CAD build for the part. Positions are in the model's coordinates, mm. Round coordinates to 2 decimals unless told otherwise and drop trailing zeros. Write each loop counter-clockwise with the first axis right and the second up, starting at its lowest first coordinate (ties: lowest second). Pieces come first, ordered by that corner, then holes. Notation, with made-up numbers: (34, -37) -> (55, -37) arc R32 ccw to (55, 0) -> close; hole circle Ø8 at (6.5, 49). An arc over 180 degrees is marked (long way). Answer in a Markdown table with one row per item. Add a question column.
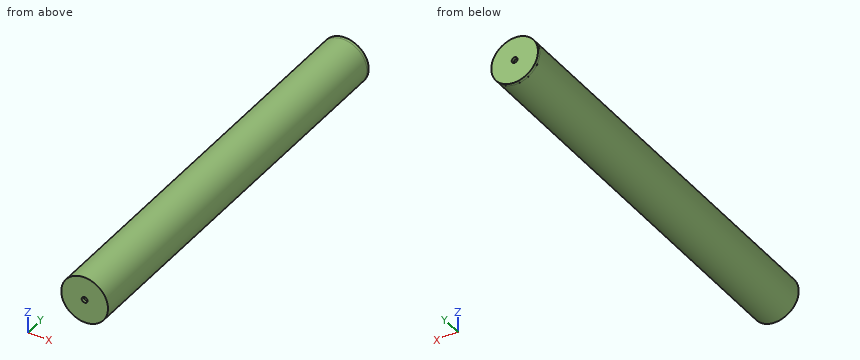
Autodesk Inventor part; units mm, degrees
ref_plane "YZ Plane" through (0, 0, 0) normal (1, 0, 0) x (0, 1, 0)
ref_plane "XZ Plane" through (0, 0, 0) normal (0, 1, 0) x (-1, 0, 0)
ref_plane "XY Plane" through (0, 0, 0) normal (0, 0, 1) x (1, 0, 0)
sketch "Sketch1" plane through (0, 0, 0) normal (0, 1, 0) x (-1, 0, 0)
  circle A0 centre (0, 0) radius 25.4
  circle A1 centre (0, 0) radius 3.175
  dimension "d0" = 50.8
  dimension "d1" = 6.35
extrude "Extrusion1" add sketch "Sketch1" along normal blind 3.175
sketch "Sketch2" plane through (0, 3.175, 0) normal (0, 1, 0) x (1, 0, 0)
  circle A0 centre (0, 0) radius 23.8125
  circle A1 centre (0, 0) radius 25.4
  dimension "d4" = 47.625
extrude "Extrusion2" add sketch "Sketch2" along normal blind 435.737
sketch "Sketch3" plane through (0, 438.912, 0) normal (0, 1, 0) x (1, 0, 0)
  circle A0 centre (0, 0) radius 25.3794
  circle A1 centre (0, 0) radius 3.175
extrude "Extrusion3" add sketch "Sketch3" along normal blind 3.175
properties part number "roller"
Item 1: Pin check, flat tips, straight feed: pin 1 (2 mm diameter, centred on y = 355, z = -7, fed in from +X); pin 2 (3 mm diameter, centred on y = 284.5, z = 11.5, fed in from -X); pin 3 (2 mm diameter, centred on x = -3, y = 166, fed in from -Z). Stop position of each tip, or through.
Item 2: Saw through at A-A on z = -13.5. Give the cut face in (x, y) (3 decimals), then the cut area to 3 significant figures.
Item 3: Saw through at B-B on y = 192.5. Give the cut face in (x, z) (1 decimal).
Item 4: Drill centre lines: probe 1 along Y at (x, z) = (-9.5, 4) (3 decimals); probe 2 along Z at (x, y) = (0, 441.15) (3 decimals); probe 3 along Z at (x, y) = (-2, 130). Where is each one in solid material? Low to high.
Recorded:
| question | item | result |
|---|---|---|
| 1 | pin 1 | x = 24.68 |
| 1 | pin 2 | x = -23.35 |
| 1 | pin 3 | z = -25.32 |
| 2 | outline | (-21.515, 0) -> (21.515, 0) -> (21.515, 438.912) -> (21.491, 438.912) -> (21.491, 442.087) -> (-21.491, 442.087) -> (-21.491, 438.912) -> (-21.515, 438.912) -> close; hole (-19.616, 3.175) -> (19.616, 3.175) -> (19.616, 438.912) -> (-19.616, 438.912) -> close |
| 2 | area | 1,930 mm2 |
| 3 | outline | circle Ø50.8 at (0, 0); hole circle Ø47.6 at (0, 0) |
| 4 | probe 1 | 0 to 3.175, 438.912 to 442.087 |
| 4 | probe 2 | -25.379 to -3.175, 3.175 to 25.379 |
| 4 | probe 3 | -25.32 to -23.73, 23.73 to 25.32 |
